Here's how the part is built. I have some questions about the finished solid (model axes, mm). Face numbers are marked on the shaded views. Give positions to 0.01 mm unless a question says otherwise; leave off trailing zeros. Order: outer loops, then holes, each group sorted by start corner. A loop starts at its lowest first (then second) coordinate and runs counter-clockwise, first axis right, second up.
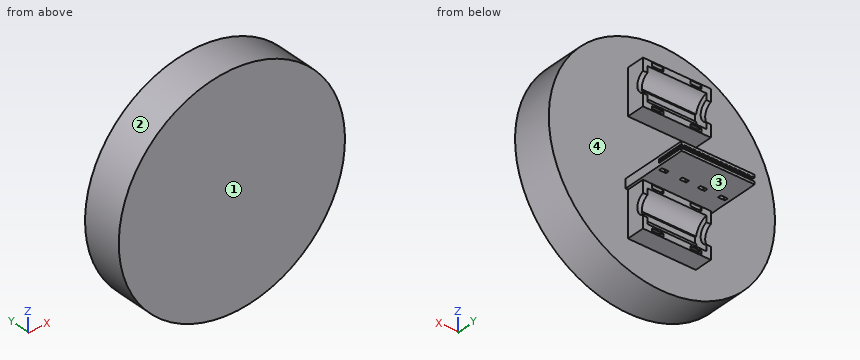
from build123d import *

# Parameters (mm, degrees)
AUFSATZ_LINEAR_AUSTRAGEN1_DEPTH      = 1.6
AUFSATZ_LINEAR_AUSTRAGEN1_DEPTH_BACK = 16.4
SKIZZE1_R                            = 50
SKIZZE2_W                            = 30
SKIZZE2_H                            = 20
AUFSATZ_LINEAR_AUSTRAGEN2_DEPTH      = 8
SKIZZE4_R                            = 7.6
SCHNITT_LINEAR_AUSTRAGEN1_DEPTH      = 85.315834812
AUFSATZ_LINEAR_AUSTRAGEN3_DEPTH      = 2
SKIZZE7_W                            = 3
SKIZZE7_H                            = 0.8
SCHNITT_LINEAR_AUSTRAGEN2_DEPTH      = 13
SKIZZE6_W                            = 5
SKIZZE6_H                            = 1.5
SPIEGELN3_COPY_1_DEPTH               = 2
SPIEGELN3_COPY_2_SKETCH_W            = 5
SPIEGELN3_COPY_2_SKETCH_H            = 1.5
SKIZZE9_W                            = 32.252572888
SKIZZE9_H                            = 4
AUFSATZ_LINEAR_AUSTRAGEN4_DEPTH      = 30
SCHNITT_LINEAR_AUSTRAGEN3_DEPTH      = 12
SKIZZE11_W                           = 1.2
SKIZZE11_H                           = 2
AUFSATZ_LINEAR_AUSTRAGEN5_DEPTH      = 20
SKIZZE13_W                           = 3
SKIZZE13_H                           = 1.2
SCHNITT_ROTATION3_ANGLE              = 180
LINEARES_MUSTER1_COUNT               = 2
LINEARES_MUSTER1_PITCH               = 9
SPIEGELN4_COPY_1_SKETCH_W            = 3
SPIEGELN4_COPY_1_SKETCH_H            = 1.2
SPIEGELN4_COPY_1_ANGLE               = 180


with BuildPart() as part:
    # Skizze1 → Aufsatz-Linear austragen1 (new, two sides: drawn at the far end of the back side and taken through both)
    with BuildSketch(Plane(origin=(0, 10, 0), x_dir=(1, 0, 0), z_dir=(0, 1, 0)).offset(-AUFSATZ_LINEAR_AUSTRAGEN1_DEPTH_BACK)):
        with Locations(Location((0, 0, 0), (0, 0, 270))):
            Circle(SKIZZE1_R)
    extrude(amount=AUFSATZ_LINEAR_AUSTRAGEN1_DEPTH + AUFSATZ_LINEAR_AUSTRAGEN1_DEPTH_BACK)

    # Skizze2 → Aufsatz-Linear austragen2 (add)
    with BuildSketch(Plane(origin=(0, 11.6, 0), x_dir=(1, 0, 0), z_dir=(0, 1, 0))):
        with Locations((0, 25.04)):
            Rectangle(SKIZZE2_W, SKIZZE2_H)
    aufsatz_linear_austragen2 = extrude(amount=AUFSATZ_LINEAR_AUSTRAGEN2_DEPTH)

    # Skizze4 → Schnitt-Linear austragen1 (cut, through all)
    with BuildSketch(Plane.ZY.offset(15)):
        with Locations((-25.04, 21.6)):
            Circle(SKIZZE4_R)
    schnitt_linear_austragen1 = extrude(amount=-SCHNITT_LINEAR_AUSTRAGEN1_DEPTH, mode=Mode.SUBTRACT)

    # Skizze5 → Aufsatz-Linear austragen3 (add)
    with BuildSketch(Plane.ZY.offset(15)):
        with BuildLine():
            Line((-29.622575695, 19.6), (-32.372121112, 19.6))
            ThreePointArc((-32.372121112, 19.6), (-25.04, 14), (-17.707878888, 19.6))
            Line((-17.707878888, 19.6), (-20.457424305, 19.6))
            ThreePointArc((-20.457424305, 19.6), (-25.04, 16.6), (-29.622575695, 19.6))
        make_face()
    aufsatz_linear_austragen3 = extrude(amount=-AUFSATZ_LINEAR_AUSTRAGEN3_DEPTH)

    # Spiegeln1: Aufsatz-Linear austragen3 across plane
    add(aufsatz_linear_austragen3.mirror(Plane(origin=(0, 0, 0), x_dir=(0, 0, 1), z_dir=(1, 0, 0))))

    # Skizze7 → Schnitt-Linear austragen2 (cut, symmetric)
    with BuildSketch(Plane(origin=(0, 0, 0), x_dir=(0, 0, -1), z_dir=(1, 0, 0))):
        with Locations((25.04, 14)):
            Rectangle(SKIZZE7_W, SKIZZE7_H)
    schnitt_linear_austragen2 = extrude(amount=SCHNITT_LINEAR_AUSTRAGEN2_DEPTH, both=True, mode=Mode.SUBTRACT)

    # Skizze6 → Schnitt-Rotation2 (revolve, cut)
    with BuildSketch(Plane.XY.offset(-25.04)):
        with Locations((-8.412172741, 30.75)):
            Rectangle(SKIZZE6_W, SKIZZE6_H)
    schnitt_rotation2 = revolve(axis=Axis((-15, 21.6, -25.04), (1, 0, 0)), mode=Mode.SUBTRACT)

    # Spiegeln2: Schnitt-Rotation2 across plane
    add(schnitt_rotation2.mirror(Plane(origin=(0, 0, 0), x_dir=(0, 0, 1), z_dir=(1, 0, 0))), mode=Mode.SUBTRACT)

    # Spiegeln3: Aufsatz-Linear austragen2, Schnitt-Linear austragen1, Aufsatz-Linear austragen3, Schnitt-Linear austragen2, Schnitt-Rotation2 across plane
    add(aufsatz_linear_austragen2.mirror(Plane.XY))
    add(schnitt_linear_austragen1.mirror(Plane.XY), mode=Mode.SUBTRACT)
    add(aufsatz_linear_austragen3.mirror(Plane.XY))
    add(schnitt_linear_austragen2.mirror(Plane.XY), mode=Mode.SUBTRACT)
    add(schnitt_rotation2.mirror(Plane.XY), mode=Mode.SUBTRACT)

    # Spiegeln3 copy 1 sketch → Spiegeln3 copy 1 (add)
    with BuildSketch(Plane(origin=(15, 0, 0), x_dir=(0, 0, -1), z_dir=(1, 0, 0))):
        with BuildLine():
            Line((-29.622575695, 19.6), (-32.372121112, 19.6))
            ThreePointArc((-32.372121112, 19.6), (-25.04, 14), (-17.707878888, 19.6))
            Line((-17.707878888, 19.6), (-20.457424305, 19.6))
            ThreePointArc((-20.457424305, 19.6), (-25.04, 16.6), (-29.622575695, 19.6))
        make_face()
    extrude(amount=-SPIEGELN3_COPY_1_DEPTH)

    # Spiegeln3 copy 2 sketch → Spiegeln3 copy 2 (revolve, cut)
    with BuildSketch(Plane(origin=(0, 0, 25.04), x_dir=(-1, 0, 0), z_dir=(0, 0, -1))):
        with Locations((-8.412172741, 30.75)):
            Rectangle(SPIEGELN3_COPY_2_SKETCH_W, SPIEGELN3_COPY_2_SKETCH_H)
    revolve(axis=Axis((15, 21.6, 25.04), (-1, 0, 0)), mode=Mode.SUBTRACT)

    # Skizze9 → Aufsatz-Linear austragen4 (add)
    with BuildSketch(Plane(origin=(0, 11.6, 0), x_dir=(1, 0, 0), z_dir=(0, 1, 0))):
        with Locations((0, 13.04)):
            Rectangle(SKIZZE9_W, SKIZZE9_H)
    extrude(amount=AUFSATZ_LINEAR_AUSTRAGEN4_DEPTH)

    # Skizze10 → Schnitt-Linear austragen3 (cut)
    with BuildSketch(Plane(origin=(0, 41.6, 0), x_dir=(1, 0, 0), z_dir=(0, 1, 0))):
        Polygon((-16.126286444, 12.215), (-14.826286444, 12.215), (-14.826286444, 13.015), (-14.126286444, 13.015), (-14.126286444, 12.215), (-12.826286444, 12.215), (-12.826286444, 13.015), (-12.126286444, 13.015), (-12.126286444, 12.215), (-10.826286444, 12.215), (-10.826286444, 13.015), (-10.126286444, 13.015), (-10.126286444, 12.215), (-8.826286444, 12.215), (-8.826286444, 13.015), (-8.126286444, 13.015), (-8.126286444, 12.215), (-6.826286444, 12.215), (-6.826286444, 13.015), (-6.126286444, 13.015), (-6.126286444, 12.215), (-4.826286444, 12.215), (-4.826286444, 13.015), (-4.126286444, 13.015), (-4.126286444, 12.215), (-2.826286444, 12.215), (-2.826286444, 13.015), (-2.126286444, 13.015), (-2.126286444, 12.215), (-0.826286444, 12.215), (-0.826286444, 13.015), (-0.126286444, 13.015), (-0.126286444, 12.215), (1.173713556, 12.215), (1.173713556, 13.015), (1.873713556, 13.015), (1.873713556, 12.215), (3.173713556, 12.215), (3.173713556, 13.015), (3.873713556, 13.015), (3.873713556, 12.215), (5.173713556, 12.215), (5.173713556, 13.015), (5.873713556, 13.015), (5.873713556, 12.215), (7.173713556, 12.215), (7.173713556, 13.015), (7.873713556, 13.015), (7.873713556, 12.215), (9.173713556, 12.215), (9.173713556, 13.015), (9.873713556, 13.015), (9.873713556, 12.215), (11.173713556, 12.215), (11.173713556, 13.015), (11.873713556, 13.015), (11.873713556, 12.215), (13.173713556, 12.215), (13.173713556, 13.015), (13.873713556, 13.015), (13.873713556, 12.215), (15.173713556, 12.215), (15.173713556, 13.015), (15.873713556, 13.015), (15.873713556, 12.215), (17.173713556, 12.215), (17.173713556, 13.865), (-16.126286444, 13.865), (-16.126286444, 13.065), align=None)
    extrude(amount=-SCHNITT_LINEAR_AUSTRAGEN3_DEPTH, mode=Mode.SUBTRACT)

    # Skizze11 → Aufsatz-Linear austragen5 (add)
    with BuildSketch(Plane(origin=(0, 11.6, 0), x_dir=(1, 0, 0), z_dir=(0, 1, 0))):
        with Locations((-10.891559468, 10.04)):
            Rectangle(SKIZZE11_W, SKIZZE11_H)
        with Locations((9.966595777, 10.04)):
            Rectangle(SKIZZE11_W, SKIZZE11_H)
    extrude(amount=AUFSATZ_LINEAR_AUSTRAGEN5_DEPTH)

    # Skizze13 → Schnitt-Rotation3 (revolve, cut)
    with BuildSketch(Plane(origin=(0, 31.1, 0), x_dir=(1, 0, 0), z_dir=(0, 1, 0))):
        with Locations((-13.026286444, 16.44)):
            Rectangle(SKIZZE13_W, SKIZZE13_H)
    schnitt_rotation3 = revolve(axis=Axis((-16.126286444, 31.1, -13.04), (-1, 0, 0)), revolution_arc=SCHNITT_ROTATION3_ANGLE, mode=Mode.SUBTRACT)

    # Lineares Muster1: Schnitt-Rotation3 ×2
    with Locations(*[(i * LINEARES_MUSTER1_PITCH, 0, 0) for i in range(1, LINEARES_MUSTER1_COUNT)]):
        add(schnitt_rotation3, mode=Mode.SUBTRACT)

    # Spiegeln4: Schnitt-Rotation3 across plane
    add(schnitt_rotation3.mirror(Plane(origin=(0, 0, 0), x_dir=(0, 0, 1), z_dir=(1, 0, 0))), mode=Mode.SUBTRACT)

    # Spiegeln4 copy 1 sketch → Spiegeln4 copy 1 (revolve, cut)
    with BuildSketch(Plane(origin=(-9, 31.1, 0), x_dir=(-1, 0, 0), z_dir=(0, 1, 0))):
        with Locations((-13.026286444, -16.44)):
            Rectangle(SPIEGELN4_COPY_1_SKETCH_W, SPIEGELN4_COPY_1_SKETCH_H)
    revolve(axis=Axis((7.126286444, 31.1, -13.04), (-1, 0, 0)), revolution_arc=SPIEGELN4_COPY_1_ANGLE, mode=Mode.SUBTRACT)


solid = part.part
Q1. I need wall thicknesses on L1, parallel to Y at x = -6.5, z = -25.5; L2, parallel to Y at x = 36.5, z = -29; L3, parallel to Z at x = -3, y = 31 (3 decimals). Which ranges of each line are inside material? Lowest first, please.
Filled sheet:
L1: y = -6.4 to 11.71, 13.21 to 13.6
L2: y = -6.4 to 11.6
L3: z = -15.04 to -13.865, -12.215 to -11.04
Q2. If we section it at A-A on y = 23: List the corners of the cut face in (x, z) for me, plus the area to 3 significant figures.
Filled sheet:
outline: (-16.13, -15.04) - (16.13, -15.04) - (16.13, -11.04) - (10.57, -11.04) - (10.57, -9.04) - (9.37, -9.04) - (9.37, -11.04) - (-10.29, -11.04) - (-10.29, -9.04) - (-11.49, -9.04) - (-11.49, -11.04) - (-16.13, -11.04) - close
area: 134 mm2
Q3. I'm going to push flat-ended pins straight in: P1, Ø1.8, axis at y = 17.5, z = -23, coming from the -X side; P2, Ø1.4, axis at x = -9.5, y = 36, coming from the -Z side; P3, Ø0.6, axis at y = 28.5, z = -13, coming from the +X side. Where does each tip first touch, or does it pass through?
Filled sheet:
P1: stops at x = -15
P2: stops at z = -15.04
P3: stops at x = 16.13
Q4. If we section it at B-B on z = 0: List the corners of the cut face in (x, y) for me.
Filled sheet:
outline: (-50, -6.4) - (50, -6.4) - (50, 11.6) - (-50, 11.6) - close
Q5. If we section it at C-C on x = -20: List the corners of the cut face in (y, z) for me, plus the area to 3 significant figures.
Filled sheet:
outline: (-6.4, -45.83) - (11.6, -45.83) - (11.6, 45.83) - (-6.4, 45.83) - close
area: 1,650 mm2
Q6. Thinking about a two-plate mould opening in Z: for the marked faces 1, 2, 3 and 4, which applies, released by +Z, released by -Z, zero draft, split by the parting line, or undercut?
Filled sheet:
face 1: zero draft
face 2: split by the parting line
face 3: released by -Z
face 4: undercut
